Source: CAD feature listing. Evaluate the final solid. Frame: model axes, mm. Round coordinates to 2 decimals unless told otherwise and drop trailing zeros. Order: outer loops, then holes, each group sorted by start corner. A loop starts at its lowest first (then second) coordinate and runs counter-clockwise, first axis right, second up.
```python
from build123d import *

# Parameters (mm, degrees)
SKETCH1_W           = 101.6
SKETCH1_H           = 254
BOSS_EXTRUDE1_DEPTH = 3.175
FILLET1_R           = 12.7
SKETCH2_W           = 19.05
SKETCH2_H           = 27.94
CUT_EXTRUDE1_DEPTH  = 137.820030058


with BuildPart() as part:
    # Sketch1 → Boss-Extrude1 (new body)
    with BuildSketch(Plane(origin=(0, 0, 0), x_dir=(1, 0, 0), z_dir=(0, 1, 0))):
        Rectangle(SKETCH1_W, SKETCH1_H)
    extrude(amount=BOSS_EXTRUDE1_DEPTH)

    # Fillet1
    fillet1_edges = [part.edges().sort_by_distance(p)[0] for p in [
        (-50.8, 1.5875, -127),
        (50.8, 1.5875, -127),
        (50.8, 1.5875, 127),
        (-50.8, 1.5875, 127),
    ]]
    fillet(fillet1_edges, radius=FILLET1_R)

    # Sketch2 → Cut-Extrude1 (cut, through all)
    with BuildSketch(Plane(origin=(0, 3.175, 0), x_dir=(1, 0, 0), z_dir=(0, 1, 0))):
        with Locations((0, -113.03)):
            Rectangle(SKETCH2_W, SKETCH2_H)
    extrude(amount=-CUT_EXTRUDE1_DEPTH, mode=Mode.SUBTRACT)


solid = part.part
```
1. Line query: line 1 along Z through (x, y) = (8.5, 1.25); line 2 along Z through (x, y) = (-40.5, 1.55). Output: solid intervals per line, ascending.
2. First-contact query: pin 1 (1.5 mm diameter, centred on x = 1, z = -94, fed in from -Y); pin 2 (1.6 mm diameter, centred on y = 1, z = 116, fed in from +X). Flat tips, straight axial feed; report the tip coordinate or a pass-through.
3. Section A-A on y = 0.8. Return loops of the section in (x, z) (3 decimals), plus the area to 3 significant figures.
4. Section B-B on x = -3. Return loops of the section in (y, z) (3 decimals).
Result:
1. line 1: z = -127 to 99.06
1. line 2: z = -126.77 to 126.77
2. pin 1: stops at y = 0
2. pin 2: stops at x = 50.77
3. outline: (-50.8, -114.3) arc R12.7 ccw to (-38.1, -127) - (38.1, -127) arc R12.7 ccw to (50.8, -114.3) - (50.8, 114.3) arc R12.7 ccw to (38.1, 127) - (9.525, 127) - (9.525, 99.06) - (-9.525, 99.06) - (-9.525, 127) - (-38.1, 127) arc R12.7 ccw to (-50.8, 114.3) - close
3. area: 25,100 mm2
4. outline: (0, -127) - (3.175, -127) - (3.175, 99.06) - (0, 99.06) - close
